```python
from build123d import *

# Parameters (mm, degrees)
SKETCH1_W           = 47.429010539
SKETCH1_H           = 22.84
BOSS_EXTRUDE1_DEPTH = 3
SKETCH2_R           = 1.25
CUT_EXTRUDE1_DEPTH  = 3


with BuildPart() as part:
    # Sketch1 → Boss-Extrude1 (new body)
    with BuildSketch(Plane.XY):
        with Locations((0.890297776, 4.627297895)):
            Rectangle(SKETCH1_W, SKETCH1_H)
    extrude(amount=BOSS_EXTRUDE1_DEPTH)

    # Sketch2 → Cut-Extrude1 (cut)
    with BuildSketch(Plane(origin=(0, 0, 0), x_dir=(-1, 0, 0), z_dir=(0, 0, -1))):
        with Locations((-0.578707914, 11.824797895)):
            Circle(SKETCH2_R)
        with Locations((13.921292086, 11.824797895)):
            Circle(SKETCH2_R)
        with BuildLine():
            Line((3.671803832, 14.669797895), (9.67078034, 14.669797895))
            Line((9.67078034, 14.669797895), (9.67078034, 12.208693547))
            ThreePointArc((9.67078034, 12.208693547), (9.784194907, 11.812134615), (10.090137637, 11.535510509))
            ThreePointArc((10.090137637, 11.535510509), (6.671292086, -3.180202105), (3.252446535, 11.535510509))
            ThreePointArc((3.252446535, 11.535510509), (3.558389265, 11.812134615), (3.671803832, 12.208693547))
            Line((3.671803832, 12.208693547), (3.671803832, 14.669797895))
        make_face()
    extrude(amount=-CUT_EXTRUDE1_DEPTH, mode=Mode.SUBTRACT)


solid = part.part
```
Source: CAD feature listing. Evaluate the final solid. Frame: model axes, mm. A direction names the side the tool comes from. Round coordinates to 2 decimals unless told otherwise and drop trailing zeros. Write each loop counter-clockwise with the first axis right and the second up, starting at its lowest first coordinate (ties: lowest second). Pieces come first, ordered by that corner, then holes. Notation, with made-up numbers: M 8.25,-24.5 L 20.25,-24.5 A25 ccw 20.25,-11.5 Z; hole C 26.25,-25 d11. An arc over 180 degrees is marked long. Use CSV: the item, a comma, the result in double quotes. Start each with the question number.
Q1. Cut plane C-C on x = -8. Output: boundary loops of the cut face in (y, z), plus the area to 3 significant figures.
Q2. Pull-direction query (X, two-part tool) for faces 3 (the face through (24.605, 4, 1)), 4 (the face through (6, 5, 3)), 5 (the face through (-7, 14.67, 1)); classes: +X half, -X half, draft (parallel to the pull), parting line (faces both ways), or undercut.
Q3. Cut plane B-B on y = 6. Output: boundary loops of the cut face in (x, z), plus the area to 3 significant figures.
Q4. Cut plane A-A on z = 0.55. Output: boundary loops of the cut face in (x, y) (3 decimals).
Q5. Line query: line 1 (X direction, y = 13.75, z = 1); line 2 (X direction, y = 11.75, z = 1.95); line 3 (X direction, y = 10.75, z = 2.55). Output: solid intervals per line, ascending. Write a range as from..to.
Q6. Access query for faces 1 (the face through (-9.671, 13, 1)), 2 (the face through (6, 5, 0)). Directions: +Z, -Z, +X, -X, +Y, -Y. A direction counts if a zero-diameter tool reaches every point of the face in a straight line with its end or side. Return the directions, or none.
Results found:
1,outline,"M -6.79,0 L -3.07,0 L -3.07,3 L -6.79,3 Z; M 14.67,0 L 16.05,0 L 16.05,3 L 14.67,3 Z"
1,area,"15.3 mm^2"
2,face 3,"+X half"
2,face 4,"draft"
2,face 5,"undercut"
3,outline,"M -22.82,0 L -14.29,0 L -14.29,3 L -22.82,3 Z; M 0.95,0 L 24.6,0 L 24.6,3 L 0.95,3 Z"
3,area,"96.5 mm^2"
4,outline,"M -22.824,-6.793 L 24.605,-6.793 L 24.605,16.047 L -22.824,16.047 Z; hole C -13.921,11.825 d2.5; hole M -10.09,11.536 A7.755 ccw long -3.252,11.536 A0.75 cw -3.672,12.209 L -3.672,14.67 L -9.671,14.67 L -9.671,12.209 A0.75 cw Z; hole C 0.579,11.825 d2.5"
5,line 1,"-22.82..-9.67, -3.67..24.6"
5,line 2,"-22.82..-15.17, -12.67..-9.83, -3.52..-0.67, 1.83..24.6"
5,line 3,"-22.82..-14.56, -13.28..-11.36, -1.98..-0.06, 1.22..24.6"
6,face 1,"+Z, -Z"
6,face 2,"-Z, +X, -X, +Y, -Y"
